The model under review builds one solid part; all positions refer to its coordinate system, in mm. Coordinates: 2 decimals unless noted, no trailing zeros. Loops run counter-clockwise (first coordinate to the right, second up) from the corner with the lowest first, then second, coordinate; pieces in that order, holes last. Notation, with made-up numbers: (-30.5, 7) - (15.5, 7) arc R10 cw to (15.5, 21) - close; hole circle Ø11 at (7.25, 43.5). An arc over 180 degrees is marked (long way). One line per item, written item: value. Start each with the question number.
1. We need section A-A, the plane y = 0. Give the boundary of the cut face in (x, z), then the cut area to 3 significant figures.
2. Insertion check: P1, Ø1, axis at y = 7.5, z = 2, coming from the -X side; P2, Ø1, axis at x = -2, z = 3, coming from the +Y side. Each pin has a flat end and moves straight along its axis. Give the tip position at first contact, or say it passes through.
3. We need section D-D, the plane z = 4. Give the boundary of the cut face in (x, y) (3 decimals), then the cut area to 3 significant figures.
4. We need section B-B, the plane y = 2.25. Give the boundary of the cut face in (x, z).
5. We need section C-C, the plane x = -1.5. Give the boundary of the cut face in (y, z).
6. Mouldability with a two-part tool opening along Y and no side actions: class faces 1 (the face through (-4.81, 2.09, 2.96)), 2 (the face through (-2.17, -9.76, 2.96)), 3 (the face through (-0.1, 2.4, 0)) as +Y half, -Y half, draft (parallel to the pull), parting line (faces both ways), or undercut.
7. To check wall thickness, follow line 1 (Y direction, x = -1, z = 2.3); line 2 (Y direction, x = 0.5, z = 0.4); line 3 (X direction, y = -0.5, z = 5.6). State the ranges of each line that lie inside material, in increasing order.
from build123d import *

# Parameters (mm, degrees)
SKETCH1_R                    = 10
SKETCH1_R_2                  = 2
BOSS_EXTRUDE1_DEPTH          = 6
F_2_05_2_05_DIAMETER_HOLE1_D = 2.05


with BuildPart() as part:
    # Sketch1 → Boss-Extrude1 (new body)
    with BuildSketch(Plane.XY):
        Circle(SKETCH1_R)
        Circle(SKETCH1_R_2, mode=Mode.SUBTRACT)
    extrude(amount=BOSS_EXTRUDE1_DEPTH)

    # Ø2.05 (2.05) Diameter Hole1 (through all)
    with Locations(Plane(origin=(-167.340510867, 18.18779669, 6.7366), x_dir=(0.05861513275015712, -0.9982806550327825, 0), z_dir=(0, 0, 1))):
        with Locations((32.447172363, 165.584185204), (25.375630841, 162.306487764), (26.072832352, 170.069471085)):
            Hole(F_2_05_2_05_DIAMETER_HOLE1_D / 2)


solid = part.part
Findings below:
1. outline: (-10, 0) - (-2, 0) - (-2, 6) - (-10, 6) - close; (2, 0) - (10, 0) - (10, 6) - (2, 6) - close
1. area: 96.0 mm2
2. P1: x = -7.14
2. P2: y = 9.89
3. outline: circle Ø20 at (0, 0); hole circle Ø2.05 at (-3.826, 2.369); hole circle Ø4 at (0, 0); hole circle Ø2.05 at (-0.139, -4.498); hole circle Ø2.05 at (3.965, 2.128)
3. area: 292 mm2
4. outline: (-9.74, 0) - (-4.84, 0) - (-4.84, 6) - (-9.74, 6) - close; (-2.81, 0) - (2.95, 0) - (2.95, 6) - (-2.81, 6) - close; (4.98, 0) - (9.74, 0) - (9.74, 6) - (4.98, 6) - close
5. outline: (-9.89, 0) - (-1.32, 0) - (-1.32, 6) - (-9.89, 6) - close; (1.32, 0) - (9.89, 0) - (9.89, 6) - (1.32, 6) - close
6. face 1: undercut
6. face 2: parting line
6. face 3: draft
7. line 1: -9.95 to -5.05, -3.94 to -1.73, 1.73 to 9.95
7. line 2: -9.99 to -5.3, -3.7 to -1.94, 1.94 to 9.99
7. line 3: -9.99 to -1.94, 1.94 to 9.99
